Here's the drawing with two shaded views (mm, measured from the low corner). I have some questions. A direction names the side the tool comes from. Coordinates: 2 decimals unless noted, no trailing zeros. Loops run counter-clockwise (first coordinate to the right, second up) from the corner with the lowest first, then second, coordinate; pieces in that order, holes last. Notation, with made-up numbers: (3.5, 9) -> (22.5, 9) arc R17 ccw to (22.5, 17) -> close; hole circle Ø8 at (74.5, 82.25). An arc over 180 degrees is marked (long way). Answer as a JSON object with one key per item and string values. Group by question number.
1) I want a section at C-C (y = 6). Write out the boundary of the cut face in (x, z).
2) I'm going to push flat-ended pins straight in: pin 1 (10 mm diameter, centred on x = 2, y = 14, fed in from -Z) (1 decimal); pin 2 (6 mm diameter, centred on y = 14, z = 14, fed in from +X); pin 3 (8 mm diameter, centred on x = 4, z = 15.5, fed in from -Y). Where does each tip first touch, or does it pass through?
3) If we mould it in two halves opening along Z, with no side actions, what happens to the marked faces 5, 6 and 7? For each: +Z half, -Z half, draft (parallel to the pull), parting line (faces both ways), or undercut.
4) I need wall thicknesses on probe 1 along Z at (x, y) = (9.5, 22); probe 2 along Z at (x, y) = (9.5, 29.6); probe 3 along Y at (x, z) = (9, 11.75). Which ranges of each line are inside material? Lowest first, please. Write a range as [from, to].
5) I want a section at D-D (y = 19.5). Write out the boundary of the cut face in (x, z).
6) Which directions (+Z, -Z, +X, -X, +Y, -Y) give clear straight access to the entire face, cutting with the end or side of a thin tool? Please do the marked faces 1, 2, 3 and 4.
7) I want a section at B-B (x = 9.5). Write out the boundary of the cut face in (y, z).
8) I want a section at A-A (z = 9.5). Write out the boundary of the cut face in (x, y), then the cut area to 3 significant figures.
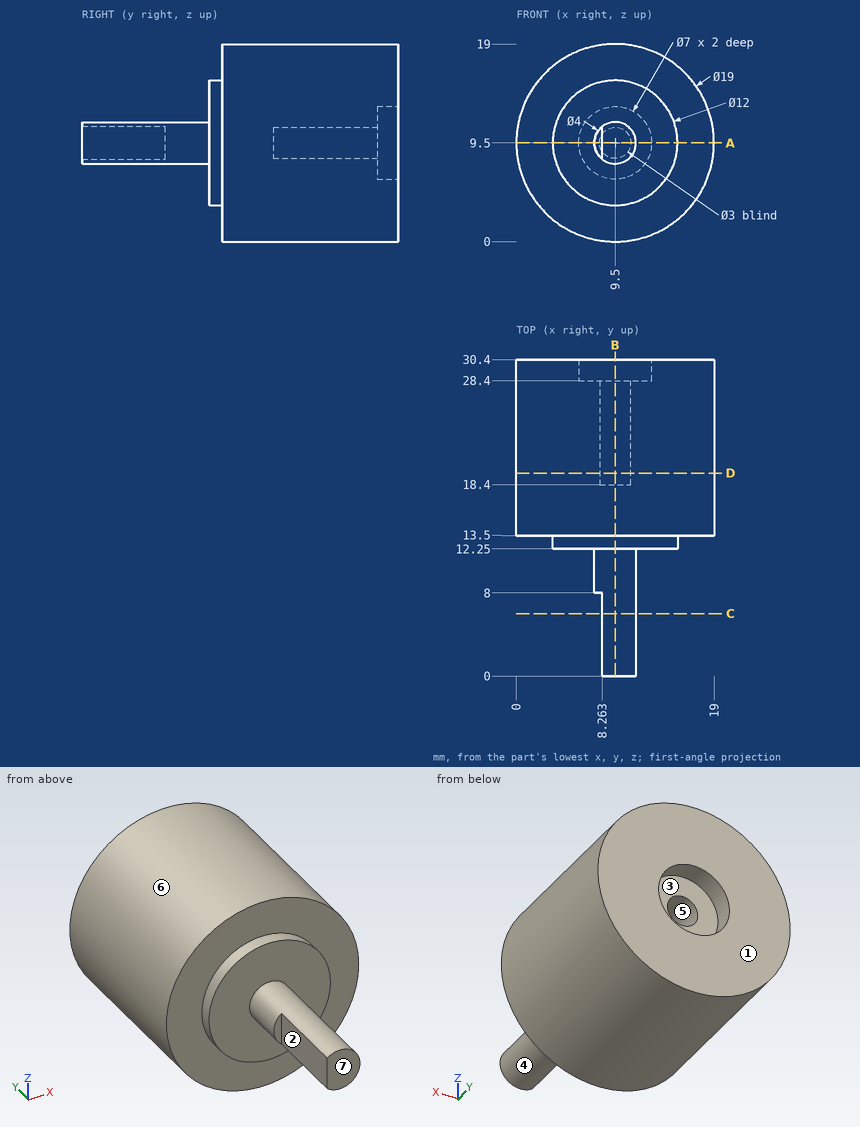
Determined:
{
 "1": {"outline": "(8.26, 7.93) arc R2 ccw (long way) to (8.26, 11.07) -> close"},
 "2": {"pin 1": "z = 0.3", "pin 2": "x = 18.88", "pin 3": "y = 12.25"},
 "3": {"face 5": "undercut", "face 6": "parting line", "face 7": "draft"},
 "4": {"probe 1": "[0, 8], [11, 19]", "probe 2": "[0, 6], [13, 19]", "probe 3": "[12.25, 28.4]"},
 "5": {"outline": "circle Ø19 at (9.5, 9.5); hole circle Ø3 at (9.5, 9.5)"},
 "6": {"face 1": "+Z, -Z, +X, -X, +Y", "face 2": "+Z, -Z, -X, -Y", "face 3": "+Y", "face 4": "-Y"},
 "7": {"outline": "(0, 7.5) -> (12.25, 7.5) -> (12.25, 3.5) -> (13.5, 3.5) -> (13.5, 0) -> (30.4, 0) -> (30.4, 6) -> (28.4, 6) -> (28.4, 8) -> (18.4, 8) -> (18.4, 11) -> (28.4, 11) -> (28.4, 13) -> (30.4, 13) -> (30.4, 19) -> (13.5, 19) -> (13.5, 15.5) -> (12.25, 15.5) -> (12.25, 11.5) -> (0, 11.5) -> close"},
 "8": {"outline": "(0, 13.5) -> (3.5, 13.5) -> (3.5, 12.25) -> (7.5, 12.25) -> (7.5, 8) -> (8.26, 8) -> (8.26, 0) -> (11.5, 0) -> (11.5, 12.25) -> (15.5, 12.25) -> (15.5, 13.5) -> (19, 13.5) -> (19, 30.4) -> (13, 30.4) -> (13, 28.4) -> (11, 28.4) -> (11, 18.4) -> (8, 18.4) -> (8, 28.4) -> (6, 28.4) -> (6, 30.4) -> (0, 30.4) -> close", "area": "335 mm^2"}
}
